CAD build for the part. Positions are in the model's coordinates, mm. A direction names the side the tool comes from. Round coordinates to 2 decimals unless told otherwise and drop trailing zeros. Write each loop counter-clockwise with the first axis right and the second up, starting at its lowest first coordinate (ties: lowest second). Pieces come first, ordered by that corner, then holes. Notation, with made-up numbers: (3, 21) - (13, 21) arc R30 ccw to (13, 54) - close; hole circle Ø10 at (37, -22.75). An arc over 180 degrees is marked (long way). Answer in a Markdown table with one row per item.
```python
from build123d import *

# Parameters (mm, degrees)
SKETCH001_R     = 1.5
POCKET_DEPTH    = 52.401
POCKET001_DEPTH = 38.701
SKETCH003_R     = 5
POCKET002_DEPTH = 10


with BuildPart() as part:
    # Sketch → Revolution (revolve)
    with BuildSketch(Plane.XY):
        Polygon((-26.2, -3.3), (-24.2, -3.3), (-23.5, -4), (-20, -4), (-19.3, -3.3), (-17.2, -3.3), (-16.5, -4), (-12.5, -4), (-12.5, -10), (12.5, -10), (12.5, -4), (16.5, -4), (17.2, -3.3), (19.3, -3.3), (20, -4), (23.5, -4), (24.2, -3.3), (26.2, -3.3), (26.2, 0), (-26.2, 0), align=None)
    revolve(axis=Axis((0, 0, 0), (1, 0, 0)))

    # Sketch001 (on Face1 of Revolution) → Pocket (cut, through all)
    with BuildSketch(Plane.YZ.offset(26.2)):
        Circle(SKETCH001_R)
    extrude(amount=-POCKET_DEPTH, mode=Mode.SUBTRACT)

    # Sketch002 (on Face16 of Pocket) → Pocket001 (cut, through all)
    with BuildSketch(Plane.YZ.offset(12.5)):
        with BuildLine():
            ThreePointArc((6, 8), (0, 10), (-6, 8))
            Line((-6, 8), (6, 8))
        make_face()
    extrude(amount=-POCKET001_DEPTH, mode=Mode.SUBTRACT)

    # Sketch003 (on Face19 of Pocket001) → Pocket002 (cut)
    with BuildSketch(Plane.XY.offset(8)):
        Circle(SKETCH003_R)
    extrude(amount=-POCKET002_DEPTH, mode=Mode.SUBTRACT)


solid = part.part
```
Q1. Saw through at D-D on z = 6.75. List the corners of the cut face in (x, y), then the cut area to 3 significant figures.
Computed:
| item | result |
|---|---|
| outline | (-12.5, -7.38) - (12.5, -7.38) - (12.5, 7.38) - (-12.5, 7.38) - close; hole circle Ø10 at (0, 0) |
| area | 290 mm2 |
Q2. Saw through at B-B on x = 0. List the corners of the cut face in (y, z), then the cut area to 3 significant figures.
Computed:
| item | result |
|---|---|
| outline | (-6, 8) arc R10 ccw (long way) to (6, 8) - (5, 8) - (5, -2) - (-5, -2) - (-5, 8) - close |
| area | 198 mm2 |
Q3. Flat gauge pins, fed straight in: pin 1 (2 mm diameter, centred on x = -12, y = -8, fed in from -Z); pin 2 (8 mm diameter, centred on x = 3.5, y = 3, fed in from +Z); pin 3 (3 mm diameter, centred on x = -13.5, z = -3.5, fed in from +Y); pin 4 (1 mm diameter, centred on y = 0.5, z = 0, fed in from +X). Where does each tip first touch, or does it go through?
Computed:
| item | result |
|---|---|
| pin 1 | stops at z = -7.14 |
| pin 2 | stops at z = 8 |
| pin 3 | stops at y = 9.71 |
| pin 4 | passes through |
Q4. Drill centre lines: line 1 (X direction, y = 0, z = 5.25); line 2 (Y direction, x = -10.25, z = 0); line 3 (Z direction, x = 20.5, y = 0). Where is each one in solid material? Low to high.
Computed:
| item | result |
|---|---|
| line 1 | x = -12.5 to -5, 5 to 12.5 |
| line 2 | y = -10 to -1.5, 1.5 to 10 |
| line 3 | z = -4 to -1.5, 1.5 to 4 |
Q5. Pull direction Y, two halves, no side cores. Call faces 1 (the cylindrical face through (15.63, -1.5, 0.07)), 2 (the flat face through (26.2, 0, -2)), 3 (the cylindrical face through (0, 0, -10)): released by +Y, released by -Y, zero draft, split by the parting line, or undercut.
Computed:
| item | result |
|---|---|
| face 1 | undercut |
| face 2 | zero draft |
| face 3 | split by the parting line |
Q6. Saw through at A-A on y = 0. Count the separate pieces of the cut face and the enclosed holes in it, then the cut area to 3 significant figures.
Computed:
| item | result |
|---|---|
| separate pieces | 3 |
| enclosed holes | 0 |
| area | 428 mm2 |
Q7. 3-axis set-ups, long thin cutter, end or side, ignore diameter. For faces 4 (the cylindrical face through (14.528, 0.867, 3.905)), 5 (the cylindrical face through (-15.33, -1.5, 0.07)), 6 (the cylindrical face through (-25.19, 2.43, -2.23)), 7 (the cylindrical face through (-18.24, 2.43, -2.23)): which of +Z, -Z, +X, -X, +Y, -Y reach the whole face in a straight line?
Computed:
| item | result |
|---|---|
| face 4 | +X |
| face 5 | +X, -X |
| face 6 | -X |
| face 7 | none |
Q8. Saw through at C-C on x = -9. List the corners of the cut face in (y, z).
Computed:
| item | result |
|---|---|
| outline | (-6, 8) arc R10 ccw (long way) to (6, 8) - close; hole circle Ø3 at (0, 0) |
